Work out the finished part from the listing and answer in its coordinate system (mm). Face numbers are marked on the shaded views. A direction names the side the tool comes from. Round coordinates to 2 decimals unless told otherwise and drop trailing zeros. Order: outer loops, then holes, each group sorted by start corner. A loop starts at its lowest first (then second) coordinate and runs counter-clockwise, first axis right, second up. Notation, with made-up numbers: (23, 80.5) -> (47, 80.5) arc R23 ccw to (47, 89.5) -> close; hole circle Ø4 at (-7.75, 4.5). An arc over 180 degrees is marked (long way). Use a Markdown table: item, result. Add a question column.
Item 1: A tool of negligible diameter and unlimited length cuts with its end or side. For the marked faces 1 and 2, from which of +Z, -Z, +X, -X, +Y, -Y can it reach the whole face along a straight path? Write none if from no direction.
Item 2: A cutting plane is placed at C-C, the plane x = 40. Determine the outline of the cut face in (y, z).
Item 3: A cutting plane is placed at A-A, the plane z = 0. Determine the outline of the cut face in (x, y).
Item 4: A cutting plane is placed at D-D, the plane x = 51. Determine the outline of the cut face in (y, z).
Item 5: For a pull along X with two mould halves and no side action, classify the marked faces 3, 4, 5 and 6 as +X half, -X half, draft (parallel to the pull), parting line (faces both ways), or undercut.
Item 6: Flat-ended cylindrical pins translate along their axes: P1, Ø10, axis at x = 24.5, z = -7.5, coming from the +Y side; P2, Ø8, axis at x = 11.5, y = 10, coming from the -Z side; P3, Ø5, axis at x = 18.5, z = -7, coming from the +Y side. Find the tip coordinate at first contact, or state that the pin passes through.
Item 7: Find the intervals of material crossed by L1, parallel to X at y = 9, z = 2; L2, parallel to Z at x = 55, y = -1; L3, parallel to Y at x = 43.5, z = 14, in increasing order. Write a range as [from, to].
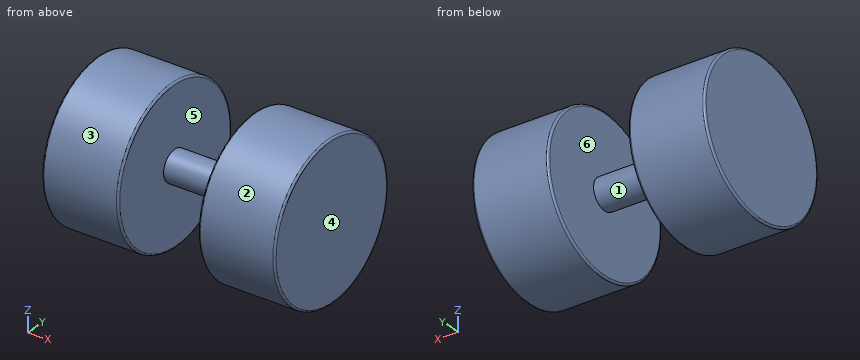
Autodesk Inventor part; units mm, degrees
ref_plane "YZ Plane" through (0, 0, 0) normal (1, 0, 0) x (0, 1, 0)
ref_plane "XZ Plane" through (0, 0, 0) normal (0, 1, 0) x (-1, 0, 0)
ref_plane "XY Plane" through (0, 0, 0) normal (0, 0, 1) x (1, 0, 0)
sketch "Náčrt1" plane through (0, 0, 0) normal (0, 0, 1) x (1, 0, 0)
  line L0 (0, 0) -> (0, -19.5)
  line L1 (0.5, -20) -> (19.5, -20)
  line L2 (20, -19.5) -> (20, 0)
  line L3 (20, 0) -> (20, -4)
  line L4 (20, -4) -> (41, -4)
  line L5 (41, -4) -> (41, -19.5)
  line L6 (41.5, -20) -> (60.5, -20)
  line L7 (61, -19.5) -> (61, 0)
  line L8 (61, 0) -> (0, 0)
  arc A0 (41, -19.5) -> (41.5, -20) centre (41.5, -19.5) ccw
  arc A1 (60.5, -20) -> (61, -19.5) centre (60.5, -19.5) ccw
  arc A2 (0, -19.5) -> (0.5, -20) centre (0.5, -19.5) ccw
  arc A3 (19.5, -20) -> (20, -19.5) centre (19.5, -19.5) ccw
  point P0 (0, -20)
  point P1 (20, -20)
  point P2 (41, -20)
  point P3 (61, -20)
  dimension "d0" = 20
  dimension "d1" = 20
  dimension "d2" = 20
  dimension "d3" = 4
  dimension "d4" = 21
  dimension "d5" = 90
  dimension "d6" = 20
  dimension "d7" = 90
  dimension "d9" = 0.5
  dimension "d10" = 0.5
revolve "Rotace1" add sketch "Náčrt1" angle 360 about axis through (61, 0, 0) along (-1, 0, 0)
properties part number "součást 2"
Reported:
| question | item | result |
|---|---|---|
| 1 | face 1 | none |
| 1 | face 2 | +X, -X |
| 2 | outline | circle Ø8 at (0, 0) |
| 3 | outline | (0, -19.5) arc R0.5 ccw to (0.5, -20) -> (19.5, -20) arc R0.5 ccw to (20, -19.5) -> (20, -4) -> (41, -4) -> (41, -19.5) arc R0.5 ccw to (41.5, -20) -> (60.5, -20) arc R0.5 ccw to (61, -19.5) -> (61, 19.5) arc R0.5 ccw to (60.5, 20) -> (41.5, 20) arc R0.5 ccw to (41, 19.5) -> (41, 4) -> (20, 4) -> (20, 19.5) arc R0.5 ccw to (19.5, 20) -> (0.5, 20) arc R0.5 ccw to (0, 19.5) -> close |
| 4 | outline | circle Ø40 at (0, 0) |
| 5 | face 3 | draft |
| 5 | face 4 | +X half |
| 5 | face 5 | undercut |
| 5 | face 6 | undercut |
| 6 | P1 | y = 19.04 |
| 6 | P2 | z = -19.08 |
| 6 | P3 | y = 19.49 |
| 7 | L1 | [0, 20], [41, 61] |
| 7 | L2 | [-19.97, 19.97] |
| 7 | L3 | [-14.28, 14.28] |
